```python
from build123d import *

# Parameters (mm, degrees)
ESQUISSE1_R             = 11
BOSS_EXTRU_1_DEPTH      = 3
ESQUISSE2_R             = 4
ESQUISSE2_R_2           = 1
ENL_V_MAT_EXTRU_1_DEPTH = 3


with BuildPart() as part:
    # Esquisse1 → Boss.-Extru.1 (new body)
    with BuildSketch(Plane.XY):
        Circle(ESQUISSE1_R)
    extrude(amount=BOSS_EXTRU_1_DEPTH)

    # Esquisse2 → Enlèv. mat.-Extru.1 (cut)
    with BuildSketch(Plane.XY.offset(3)):
        Circle(ESQUISSE2_R)
        with Locations((0, 8)):
            Circle(ESQUISSE2_R_2)
        with Locations((0, -8)):
            Circle(ESQUISSE2_R_2)
        with Locations((8, 0)):
            Circle(ESQUISSE2_R_2)
        with Locations((-8, 0)):
            Circle(ESQUISSE2_R_2)
    extrude(amount=-ENL_V_MAT_EXTRU_1_DEPTH, mode=Mode.SUBTRACT)


solid = part.part
```
Work out the finished part from the listing and answer in its coordinate system (mm). Round coordinates to 2 decimals unless told otherwise and drop trailing zeros. Write each loop counter-clockwise with the first axis right and the second up, starting at its lowest first coordinate (ties: lowest second). Pieces come first, ordered by that corner, then holes.
1) Flat-ended cylindrical pins translate along their axes: P1, Ø2, axis at x = 3, y = -6, coming from the -Z side; P2, Ø1.2, axis at x = 0, y = -8, coming from the +Z side; P3, Ø1.5, axis at x = -4, z = 1, coming from the +Y side. Find the tip coordinate at first contact, or state that the pin passes through.
2) Consider probe 1 along Y at (x, z) = (0, 1.7); probe 2 along X at (y, z) = (-0.5, 2); probe 3 along Y at (x, z) = (-1.75, 2.05). Determine where each line is inside the solid, lowest interval first.
3) A cutting plane is placed at A-A on y = 0. Determine the outline of the cut face in (x, z).
4) A cutting plane is placed at C-C on z = 2.5. Determine the outline of the cut face in (x, y).
5) A cutting plane is placed at D-D on y = 8.5. Determine the outline of the cut face in (x, z), and give its area (3 significant figures).
6) Determine the mould class of faces 1 (the face through (0, -7, 2)), 2 (the face through (-2.38, -10.74, 1.48)), 3 (the face through (0, -5, 3)) for opening direction X: pulls with the +X half, pulls with the -X half, needs draft (parallel to the pull), parting line crosses it, or undercut.
Entries:
1. P1: stops at z = 0
1. P2: passes through
1. P3: stops at y = 10.51
2. probe 1: y = -11 to -9, -7 to -4, 4 to 7, 9 to 11
2. probe 2: x = -10.99 to -8.87, -7.13 to -3.97, 3.97 to 7.13, 8.87 to 10.99
2. probe 3: y = -10.86 to -3.6, 3.6 to 10.86
3. outline: (-11, 0) - (-9, 0) - (-9, 3) - (-11, 3) - close; (-7, 0) - (-4, 0) - (-4, 3) - (-7, 3) - close; (4, 0) - (7, 0) - (7, 3) - (4, 3) - close; (9, 0) - (11, 0) - (11, 3) - (9, 3) - close
4. outline: circle Ø22 at (0, 0); hole circle Ø2 at (-8, 0); hole circle Ø8 at (0, 0); hole circle Ø2 at (0, -8); hole circle Ø2 at (0, 8); hole circle Ø2 at (8, 0)
5. outline: (-6.98, 0) - (-0.87, 0) - (-0.87, 3) - (-6.98, 3) - close; (0.87, 0) - (6.98, 0) - (6.98, 3) - (0.87, 3) - close
5. area: 36.7 mm2
6. face 1: undercut
6. face 2: parting line crosses it
6. face 3: needs draft
